Design review of the part built by this model. Coordinates are the model's own, in mm. Face numbers are marked on the shaded views. A direction names the side the tool comes from. Give positions to 0.01 mm unless a question says otherwise; leave off trailing zeros. Order: outer loops, then holes, each group sorted by start corner. A loop starts at its lowest first (then second) coordinate and runs counter-clockwise, first axis right, second up. Notation, with made-up numbers: (63.25, -7.5) -> (122.25, -7.5) arc R18 cw to (122.25, 13.5) -> close; hole circle Ø5 at (1.5, -29). An arc over 180 degrees is marked (long way). Return JSON: item names as keys, results as strings.
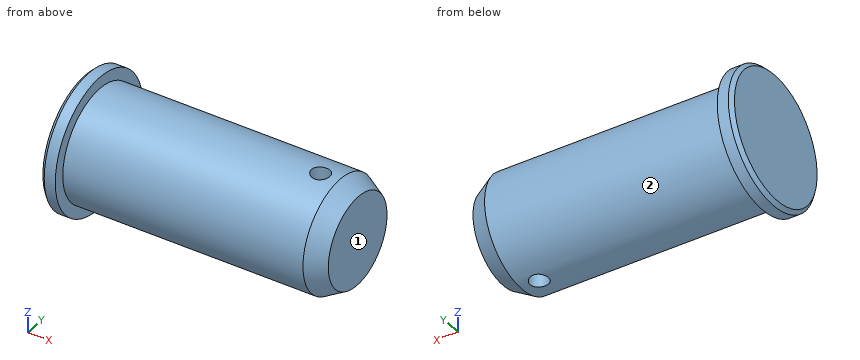
```python
from build123d import *

# Parameters (mm, degrees)
CHAMFER_1_SIZE      = 2
SKETCH_2_R          = 5
CUT_EXTRUDE_1_DEPTH = 171.553510665


with BuildPart() as part:
    # 草图1 → 旋转1 (revolve)
    with BuildSketch(Plane.XY, mode=Mode.PRIVATE) as revolve_1_sk:
        Polygon((0, 0), (0, 36.5), (8, 36.5), (8, 30.25), (138, 30.25), (148, 24.5), (148, 0), align=None)
    revolve(revolve_1_sk.sketch.rotate(Axis((0, 0, 0), (1, 0, 0)), 90), axis=Axis((0, 0, 0), (1, 0, 0)))

    # 倒角1
    chamfer_1_edges = [part.edges().sort_by_distance(p)[0] for p in [
        (0, 0, -36.5),
    ]]
    chamfer(chamfer_1_edges, length=CHAMFER_1_SIZE)

    # 草图2 → 切除-拉伸1 (cut, through all)
    with BuildSketch(Plane.XY.offset(40)):
        with Locations((128, 0)):
            Circle(SKETCH_2_R)
    extrude(amount=-CUT_EXTRUDE_1_DEPTH, mode=Mode.SUBTRACT)


solid = part.part
```
Item 1: Add section B-B (z = 0). Give the boundary of the cut face in (x, y), plus the area to 3 significant figures.
Result set:
{"outline": "(0, -34.5) -> (2, -36.5) -> (8, -36.5) -> (8, -30.25) -> (138, -30.25) -> (148, -24.5) -> (148, 24.5) -> (138, 30.25) -> (8, 30.25) -> (8, 36.5) -> (2, 36.5) -> (0, 34.5) -> close; hole circle Ø10 at (128, 0)", "area": "8,910 mm^2"}
Item 2: Add section C-C (x = 68). Give the boundary of the cut face in (y, z), plus the area to 3 significant figures.
Result set:
{"outline": "circle Ø60.5 at (0, 0)", "area": "2,870 mm^2"}
Item 3: For pin 1 (1 mm diameter, centred on y = 5, z = -25, fed in from +X); pin 2 (8 mm diameter, centred on x = 128, y = 0, fed in from +Z); pin 3 (2 mm diameter, centred on x = 106, y = 9.5, fed in from -Z); pin 4 (10 mm diameter, centred on x = 50.5, z = -18.5, fed in from -Y), all flat-tipped, find the tip position at first contact; note any pin that passes through.
Result set:
{"pin 1": "stops at x = 147.14", "pin 2": "passes through", "pin 3": "stops at z = -29.03", "pin 4": "stops at y = -27.07"}
Item 4: Wall thickness on L1, parallel to X at y = 0, z = -1.5; L2, parallel to X at y = 18, z = -26; L3, parallel to Y at x = 128, z = -14: over which ranges is each line inside the solid? List them lowest first. Write a range as [from, to].
Result set:
{"L1": "x = [0, 123], [133, 148]", "L2": "x = [0, 8]", "L3": "y = [-26.82, -5], [5, 26.82]"}
Item 5: Add section A-A (y = 0). Give the boundary of the cut face in (x, z), plus the area to 3 significant figures.
Result set:
{"outline": "(0, -34.5) -> (2, -36.5) -> (8, -36.5) -> (8, -30.25) -> (123, -30.25) -> (123, 30.25) -> (8, 30.25) -> (8, 36.5) -> (2, 36.5) -> (0, 34.5) -> close; (133, -30.25) -> (138, -30.25) -> (148, -24.5) -> (148, 24.5) -> (138, 30.25) -> (133, 30.25) -> close", "area": "8,390 mm^2"}
Item 6: Machinability: for the marked faces 1 and 2, which of the approach directions +Z, -Z, +X, -X, +Y, -Y give a long, thin tool a straight path to every point of the face, cutting with its end or side? Answer none if there is none.
Result set:
{"face 1": "+Z, -Z, +X, +Y, -Y", "face 2": "+X"}
